Design review of the part built by this model. Coordinates are the model's own, in mm. Coordinates: 2 decimals unless noted, no trailing zeros. Write each loop counter-clockwise with the first axis right and the second up, starting at its lowest first coordinate (ties: lowest second). Pieces come first, ordered by that corner, then holes. Notation, with made-up numbers: (6, 50) - (42, 50) arc R19 cw to (42, 79) - close; hole circle Ø8 at (15, 48). An arc over 180 degrees is marked (long way). Answer as a JSON object with one key per item and string values.
```python
from build123d import *

# Parameters (mm, degrees)
SKETCH1_R           = 1.5
BOSS_EXTRUDE1_DEPTH = 3.175


with BuildPart() as part:
    # Sketch1 → Boss-Extrude1 (new body)
    with BuildSketch(Plane(origin=(0, 0, 0), x_dir=(1, 0, 0), z_dir=(0, 1, 0))):
        Polygon((-25.4, 10.621890813), (-25.4, -11.476109187), (-11.476109187, -25.4), (10.621890813, -25.4), (25.4, -10.621890813), (25.4, 11.476109187), (11.476109187, 25.4), (-10.621890813, 25.4), align=None)
        with Locations((-17.78, 5.969)):
            Circle(SKETCH1_R, mode=Mode.SUBTRACT)
        with Locations((-17.78, -5.969)):
            Circle(SKETCH1_R, mode=Mode.SUBTRACT)
        with Locations((-5.969, 17.78)):
            Circle(SKETCH1_R, mode=Mode.SUBTRACT)
        with Locations((5.969, 17.78)):
            Circle(SKETCH1_R, mode=Mode.SUBTRACT)
        with Locations((17.78, 5.969)):
            Circle(SKETCH1_R, mode=Mode.SUBTRACT)
        with Locations((17.78, -5.969)):
            Circle(SKETCH1_R, mode=Mode.SUBTRACT)
        with Locations((5.969, -17.78)):
            Circle(SKETCH1_R, mode=Mode.SUBTRACT)
        with Locations((-5.969, -17.78)):
            Circle(SKETCH1_R, mode=Mode.SUBTRACT)
        with BuildLine():
            Line((-24.13, -8.047109187), (-24.13, 7.192890813))
            ThreePointArc((-24.13, 7.192890813), (-22.86, 8.462890813), (-21.59, 7.192890813))
            Line((-21.59, 7.192890813), (-21.59, -8.047109187))
            ThreePointArc((-21.59, -8.047109187), (-22.86, -9.317109187), (-24.13, -8.047109187))
        make_face(mode=Mode.SUBTRACT)
        with BuildLine():
            Line((-20.956600881, 9.576269931), (-10.180293536, 20.352577276))
            ThreePointArc((-10.180293536, 20.352577276), (-10.180293536, 22.1486285), (-11.97634476, 22.1486285))
            Line((-11.97634476, 22.1486285), (-22.752652105, 11.372321155))
            ThreePointArc((-22.752652105, 11.372321155), (-22.752652105, 9.576269931), (-20.956600881, 9.576269931))
        make_face(mode=Mode.SUBTRACT)
        with BuildLine():
            Line((-8.047109187, 21.59), (7.192890813, 21.59))
            ThreePointArc((7.192890813, 21.59), (8.462890813, 22.86), (7.192890813, 24.13))
            Line((7.192890813, 24.13), (-8.047109187, 24.13))
            ThreePointArc((-8.047109187, 24.13), (-9.317109187, 22.86), (-8.047109187, 21.59))
        make_face(mode=Mode.SUBTRACT)
        with BuildLine():
            Line((9.576269931, 20.956600881), (20.352577276, 10.180293536))
            ThreePointArc((20.352577276, 10.180293536), (22.1486285, 10.180293536), (22.1486285, 11.97634476))
            Line((22.1486285, 11.97634476), (11.372321155, 22.752652105))
            ThreePointArc((11.372321155, 22.752652105), (9.576269931, 22.752652105), (9.576269931, 20.956600881))
        make_face(mode=Mode.SUBTRACT)
        with BuildLine():
            Line((21.59, 8.047109187), (21.59, -7.192890813))
            ThreePointArc((21.59, -7.192890813), (22.86, -8.462890813), (24.13, -7.192890813))
            Line((24.13, -7.192890813), (24.13, 8.047109187))
            ThreePointArc((24.13, 8.047109187), (22.86, 9.317109187), (21.59, 8.047109187))
        make_face(mode=Mode.SUBTRACT)
        with BuildLine():
            Line((20.956600881, -9.576269931), (10.180293536, -20.352577276))
            ThreePointArc((10.180293536, -20.352577276), (10.180293536, -22.1486285), (11.97634476, -22.1486285))
            Line((11.97634476, -22.1486285), (22.752652105, -11.372321155))
            ThreePointArc((22.752652105, -11.372321155), (22.752652105, -9.576269931), (20.956600881, -9.576269931))
        make_face(mode=Mode.SUBTRACT)
        with BuildLine():
            Line((8.047109187, -21.59), (-7.192890813, -21.59))
            ThreePointArc((-7.192890813, -21.59), (-8.462890813, -22.86), (-7.192890813, -24.13))
            Line((-7.192890813, -24.13), (8.047109187, -24.13))
            ThreePointArc((8.047109187, -24.13), (9.317109187, -22.86), (8.047109187, -21.59))
        make_face(mode=Mode.SUBTRACT)
        with BuildLine():
            Line((-9.576269931, -20.956600881), (-20.352577276, -10.180293536))
            ThreePointArc((-20.352577276, -10.180293536), (-22.1486285, -10.180293536), (-22.1486285, -11.97634476))
            Line((-22.1486285, -11.97634476), (-11.372321155, -22.752652105))
            ThreePointArc((-11.372321155, -22.752652105), (-9.576269931, -22.752652105), (-9.576269931, -20.956600881))
        make_face(mode=Mode.SUBTRACT)
    extrude(amount=BOSS_EXTRUDE1_DEPTH)


solid = part.part
```
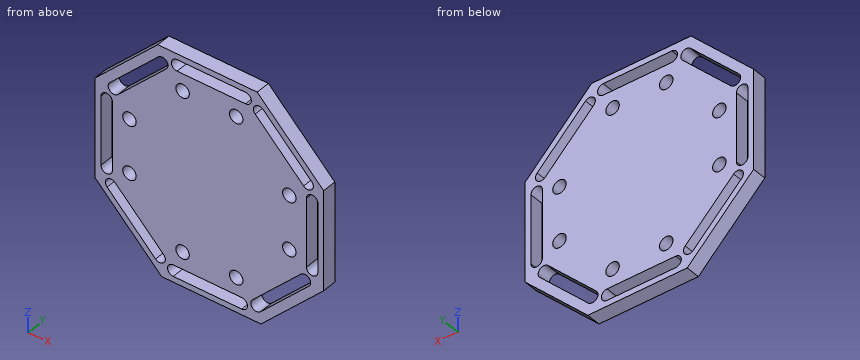
(1) To check wall thickness, follow line 1 (X direction, y = 1.2, z = -6); line 2 (Z direction, x = -2, y = 2.8). State the ranges of each line that lie inside material, in increasing order. Write a range as from..to.
Solved:
{"line 1": "x = -25.4..-24.13, -21.59..-19.28, -16.28..16.28, 19.28..21.59, 24.13..25.4", "line 2": "z = -25.4..-24.13, -21.59..21.59, 24.13..25.4"}
(2) Take a section at A-A, the plane x = 17.78. Write out the cut boundary in (y, z) (3 decimals).
Solved:
{"outline": "(0, -19.096) - (3.175, -19.096) - (3.175, -16.345) - (0, -16.345) - close; (0, -12.753) - (3.175, -12.753) - (3.175, -7.469) - (0, -7.469) - close; (0, -4.469) - (3.175, -4.469) - (3.175, 4.469) - (0, 4.469) - close; (0, 7.469) - (3.175, 7.469) - (3.175, 12.753) - (0, 12.753) - close; (0, 16.345) - (3.175, 16.345) - (3.175, 18.242) - (0, 18.242) - close"}
(3) Take a section at B-B, the plane z = 18.5. Write out the cut boundary in (x, y) (3 decimals).
Solved:
{"outline": "(-18.376, 0) - (-15.625, 0) - (-15.625, 3.175) - (-18.376, 3.175) - close; (-12.033, 0) - (-7.285, 0) - (-7.285, 3.175) - (-12.033, 3.175) - close; (-4.653, 0) - (4.653, 0) - (4.653, 3.175) - (-4.653, 3.175) - close; (7.285, 0) - (12.033, 0) - (12.033, 3.175) - (7.285, 3.175) - close; (15.625, 0) - (17.522, 0) - (17.522, 3.175) - (15.625, 3.175) - close"}
(4) For pin 1 (1.8 mm diameter, centred on x = 5.969, z = 17.78, fed in from +Y), flat-tipped, find the tip position at first contact; note if it passes through.
Solved:
{"pin 1": "passes through"}
(5) Take a section at C-C, the plane z = 2.5. Write out the cut boundary in (x, y) (3 decimals), and give its area (3 significant figures).
Solved:
{"outline": "(-25.4, 0) - (-24.13, 0) - (-24.13, 3.175) - (-25.4, 3.175) - close; (-21.59, 0) - (21.59, 0) - (21.59, 3.175) - (-21.59, 3.175) - close; (24.13, 0) - (25.4, 0) - (25.4, 3.175) - (24.13, 3.175) - close", "area": "145 mm^2"}
(6) Take a section at D-D, the plane y = 2.45. Give the number of separate pieces and of enclosed holes in the cut face, and give its area (3 significant figures).
Solved:
{"separate pieces": "1", "enclosed holes": "16", "area": "1,760 mm^2"}
